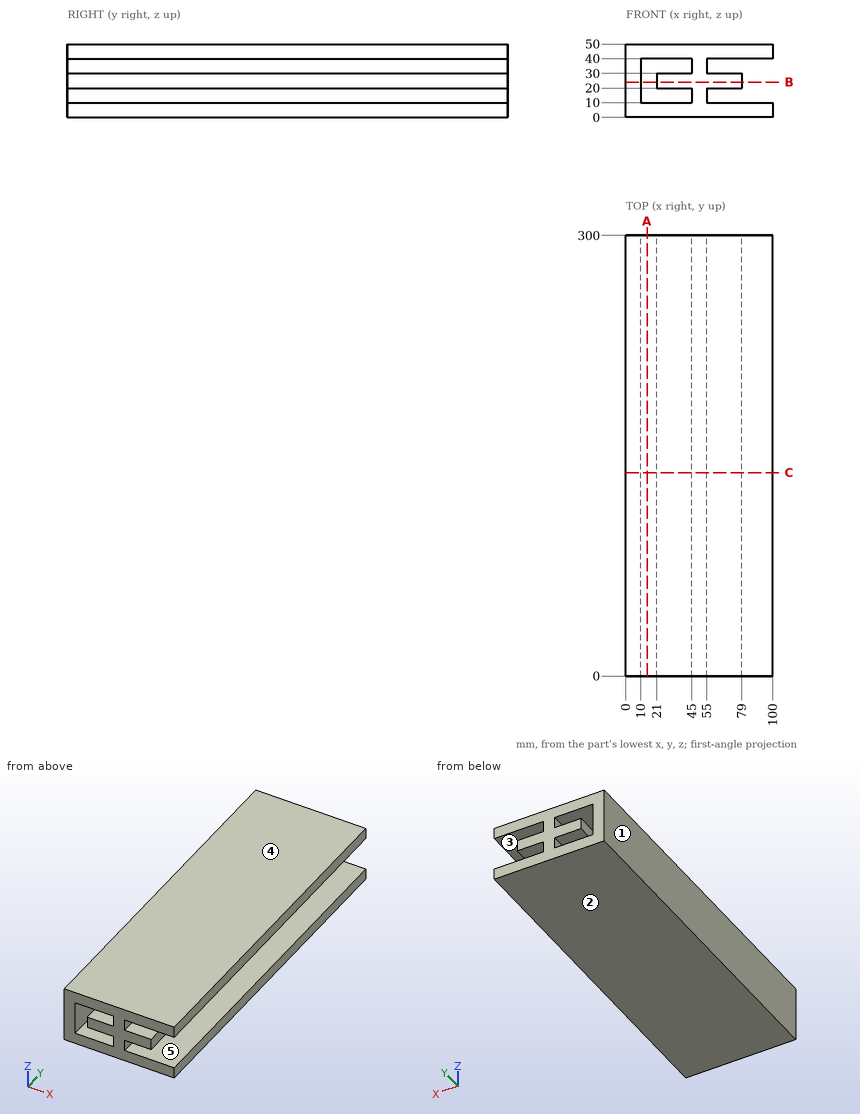
Geometry: see drawing. Coordinates: mm, zero at the bounding-box minimum. A direction names the side the tool comes from. Coordinates: 2 decimals unless noted, no trailing zeros. Write each loop counter-clockwise with the first axis right and the second up, starting at its lowest first coordinate (ties: lowest second). Pieces come first, ordered by that corner, then holes. Notation, with made-up numbers: (-24.75, 38.25) - (27.25, 38.25) arc R21 cw to (27.25, 51.25) - close; hole circle Ø11 at (-40, -21.75). An arc over 180 degrees is marked (long way). Put each result on its own line as item: value. Start each with the question number.
1) Contact query for flat-ended pins moving along their axis: pin 1 (3 mm diameter, centred on y = 244.5, z = 31, fed in from +X); pin 2 (2 mm diameter, centred on y = 237.5, z = 16, fed in from +X). Output: stop coordinate, or through.
2) Cut plane B-B (z = 24). Return the cut outline in (x, y), plus the area to 3 significant figures.
3) Cut plane A-A (x = 14.5). Return the cut outline in (y, z), plus the area to 3 significant figures.
4) Cut plane C-C (y = 138.5). Return the cut outline in (x, z), plus the area to 3 significant figures.
5) Mould query, pull axis Z, two halves, no side actions, for the marked faces 1, 2 and 3. Classes: pulls with the +Z half, pulls with the -Z half, needs draft (parallel to the pull), parting line crosses it, or undercut.
6) Reachability of the marked faces 4 and 5 from +Z, -Z, +X, -X, +Y, -Y: full face, straight path, thin tool, end or side. Return the list, or none.
7) Ray query, L1, parallel to Z at x = 31, y = 95; L2, parallel to X at y = 46.5, z = 22; L3, parallel to Z at x = 81, y = 126.5. Return the intervals inside material, ascending.
Resolved:
1. pin 1: stops at x = 79
1. pin 2: stops at x = 55
2. outline: (0, 0) - (10, 0) - (10, 300) - (0, 300) - close; (21, 0) - (79, 0) - (79, 300) - (21, 300) - close
2. area: 20,400 mm2
3. outline: (0, 0) - (300, 0) - (300, 10) - (0, 10) - close; (0, 40) - (300, 40) - (300, 50) - (0, 50) - close
3. area: 6,000 mm2
4. outline: (0, 0) - (100, 0) - (100, 10) - (55, 10) - (55, 20) - (79, 20) - (79, 30) - (55, 30) - (55, 40) - (100, 40) - (100, 50) - (0, 50) - close; hole (10, 10) - (45, 10) - (45, 20) - (21, 20) - (21, 30) - (45, 30) - (45, 40) - (10, 40) - close
4. area: 3,080 mm2
5. face 1: needs draft
5. face 2: pulls with the -Z half
5. face 3: undercut
6. face 4: +Z, +X, -X, +Y, -Y
6. face 5: +X, +Y, -Y
7. L1: z = 0 to 10, 20 to 30, 40 to 50
7. L2: x = 0 to 10, 21 to 79
7. L3: z = 0 to 10, 40 to 50
